Part model, mm, in its own coordinate system. Face numbers are marked on the shaded views. A direction names the side the tool comes from. Round coordinates to 2 decimals unless told otherwise and drop trailing zeros. Order: outer loops, then holes, each group sorted by start corner. A loop starts at its lowest first (then second) coordinate and runs counter-clockwise, first axis right, second up. Notation, with made-up numbers: (89.5, -29.5) - (146.5, -29.5) arc R12 ccw to (146.5, -14.5) - close; hole circle Ø2 at (57.25, 33). An arc over 180 degrees is marked (long way). Return JSON: item names as keys, results as strings. Group by question number.
Item 1: Two-plate mould, pull along X, no slides. Class the marked faces 3, 4, 5 and 6: released by +X, released by -X, zero draft, split by the parting line, or undercut.
Item 2: Saw through at A-A on z = -17.5. List the corners of the cut face in (x, y).
Item 3: Saw through at D-D on x = -8. List the corners of the cut face in (y, z).
Item 4: Tool access for the marked faces 1 and 2: list every direction of +Z, -Z, +X, -X, +Y, -Y with a clear straight run to the whole face (end or side of a thin tool).
Item 5: Saw through at C-C on x = 0. List the corners of the cut face in (y, z), and give its area (3 significant figures).
Item 6: Saw through at B-B on x = 15.5. List the corners of the cut face in (y, z).
Item 7: Probe probe 1 along Y at (x, z) = (0, 22.15); probe 2 along X at (y, z) = (26, -5.5); probe 3 along Z at (x, y) = (-29.5, 53). List the from-to ranges inside material, lowest first.
Item 8: Drop a flat-ended pin along its axis: pin 1 (10 mm diameter, centred on x = 9.5, z = -14.5, fed in from +Y). Give the stop position or say it passes through.
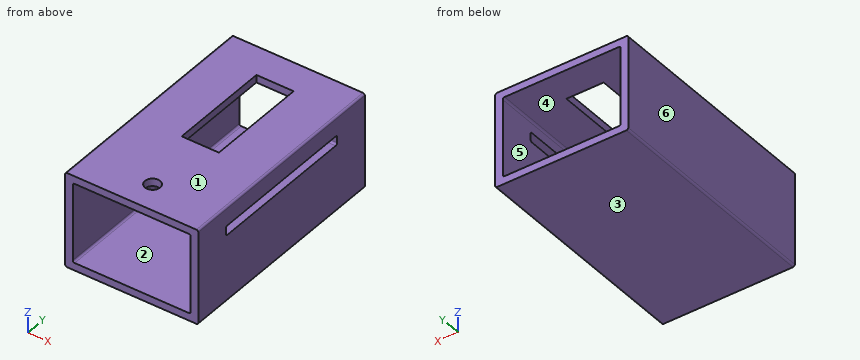
Autodesk Fusion 360 part; units mm, degrees
sketch "Sketch1" plane through (0, 0, 0) normal (0, 1, 0) x (1, 0, 0)
  line L0 (-65, 0) -> (50, 0) construction
  line L1 (-34, -25) -> (34, -25)
  line L2 (35, -24) -> (35, 24)
  line L3 (34, 25) -> (-34, 25)
  line L4 (-35, 24) -> (-35, -24)
  line L5 (-35, 25) -> (35, -25) construction
  line L6 (-35, -25) -> (35, 25) construction
  arc A0 (-35, -24) -> (-34, -25) centre (-34, -24) ccw
  arc A1 (34, -25) -> (35, -24) centre (34, -24) ccw
  arc A2 (35, 24) -> (34, 25) centre (34, 24) ccw
  arc A3 (-34, 25) -> (-35, 24) centre (-34, 24) ccw
  point P0 (-32.7786, 20)
  point P1 (32.2214, 20)
  point P2 (-32.7786, -20)
  dimension "d7" = 70
  dimension "d8" = 50
  dimension "d9" = 1
  dimension "d10" = 1
extrude "Extrude1" add sketch "Sketch1" along normal mid plane 120
sketch "Sketch2" plane through (0, -60, 0) normal (0, -1, 0) x (1, 0, 0)
  arc A0 (-35, -24) -> (-34, -25) centre (-34, -24) ccw
  line L0 (-34, -25) -> (34, -25)
  arc A1 (34, -25) -> (35, -24) centre (34, -24) ccw
  line L1 (35, -24) -> (35, 24)
  arc A2 (35, 24) -> (34, 25) centre (34, 24) ccw
  line L2 (34, 25) -> (-34, 25)
  arc A3 (-34, 25) -> (-35, 24) centre (-34, 24) ccw
  line L3 (-35, 24) -> (-35, -24)
  line L4 (-29.9936, -20.9993) -> (29.9936, -20.9993)
  line L5 (30.9936, -19.9993) -> (30.9936, 19.9993)
  line L6 (29.9936, 20.9993) -> (-29.9936, 20.9993)
  line L7 (-30.9936, 19.9993) -> (-30.9936, -19.9993)
  arc A4 (-29.9936, 20.9993) -> (-30.9936, 19.9993) centre (-29.9936, 19.9993) ccw
  arc A5 (30.9936, 19.9993) -> (29.9936, 20.9993) centre (29.9936, 19.9993) ccw
  arc A6 (29.9936, -20.9993) -> (30.9936, -19.9993) centre (29.9936, -19.9993) ccw
  arc A7 (-30.9936, -19.9993) -> (-29.9936, -20.9993) centre (-29.9936, -19.9993) ccw
  line L8 (-45, 0) -> (50, 0) construction
  line L9 (0, 30) -> (0, -30) construction
  dimension "d11" = 1
extrude "Extrude2" cut sketch "Sketch2" against normal blind 120 contours L4 L5 L6 L7 A4 A5 A6 A7
sketch "Sketch3" plane through (0, 0, 25) normal (0, 0, 1) x (-1, 0, 0)
  line L0 (-34, 60) -> (-34, -60)
  line L1 (-34, -60) -> (34, -60)
  line L2 (34, -60) -> (34, 60)
  line L3 (34, 60) -> (-34, 60)
  circle A0 centre (0, 45) radius 4
  line L4 (10, 10.3084) -> (-9.5736, 10.3084)
  line L5 (-9.5736, 10.3084) -> (-9.5736, -43.5288)
  line L6 (-9.5736, -43.5288) -> (10, -43.5288)
  line L7 (10, -43.5288) -> (10, 10.3084)
  dimension "d14" = 8
extrude "Extrude3" cut sketch "Sketch3" against normal blind 5 contours A0 | L4 L5 L6 L7
sketch "Sketch4" plane through (35, 0, 0) normal (1, 0, 0) x (0, 1, 0)
  line L0 (-60, -24) -> (60, -24)
  line L1 (60, -24) -> (60, 24)
  line L2 (60, 24) -> (-60, 24)
  line L3 (-60, 24) -> (-60, -24)
  line L4 (-39, 15) -> (39, 15)
  line L5 (40, 14) -> (40, 11)
  line L6 (39, 10) -> (-39, 10)
  line L7 (-40, 11) -> (-40, 14)
  arc A0 (-39, 15) -> (-40, 14) centre (-39, 14) ccw
  arc A1 (40, 14) -> (39, 15) centre (39, 14) ccw
  arc A2 (39, 10) -> (40, 11) centre (39, 11) ccw
  arc A3 (-40, 11) -> (-39, 10) centre (-39, 11) ccw
  dimension "d17" = 1
extrude "Extrude4" cut sketch "Sketch4" against normal blind 5 contours L4 L5 L6 L7 A0 A1 A2 A3
Filled in:
{
 "1": {"face 3": "zero draft", "face 4": "undercut", "face 5": "undercut", "face 6": "released by -X"},
 "2": {"outline": "(-35, -60) - (-30.99, -60) - (-30.99, 60) - (-35, 60) - close; (30.99, -60) - (35, -60) - (35, 60) - (30.99, 60) - close"},
 "3": {"outline": "(-60, -25) - (60, -25) - (60, -21) - (-60, -21) - close; (-60, 21) - (-10.31, 21) - (-10.31, 25) - (-60, 25) - close; (43.53, 21) - (60, 21) - (60, 25) - (43.53, 25) - close"},
 "4": {"face 1": "+Z, +X, -X, +Y, -Y", "face 2": "+Y, -Y"},
 "5": {"outline": "(-60, -25) - (60, -25) - (60, -21) - (-60, -21) - close; (-60, 21) - (-49, 21) - (-49, 25) - (-60, 25) - close; (-41, 21) - (-10.31, 21) - (-10.31, 25) - (-41, 25) - close; (43.53, 21) - (60, 21) - (60, 25) - (43.53, 25) - close", "area": "713 mm^2"},
 "6": {"outline": "(-60, -25) - (60, -25) - (60, -21) - (-60, -21) - close; (-60, 21) - (60, 21) - (60, 25) - (-60, 25) - close"},
 "7": {"probe 1": "y = -60 to -49, -41 to -10.31, 43.53 to 60", "probe 2": "x = -35 to -30.99, 30.99 to 35", "probe 3": "z = -25 to -21, 21 to 25"},
 "8": {"pin 1": "passes through"}
}
